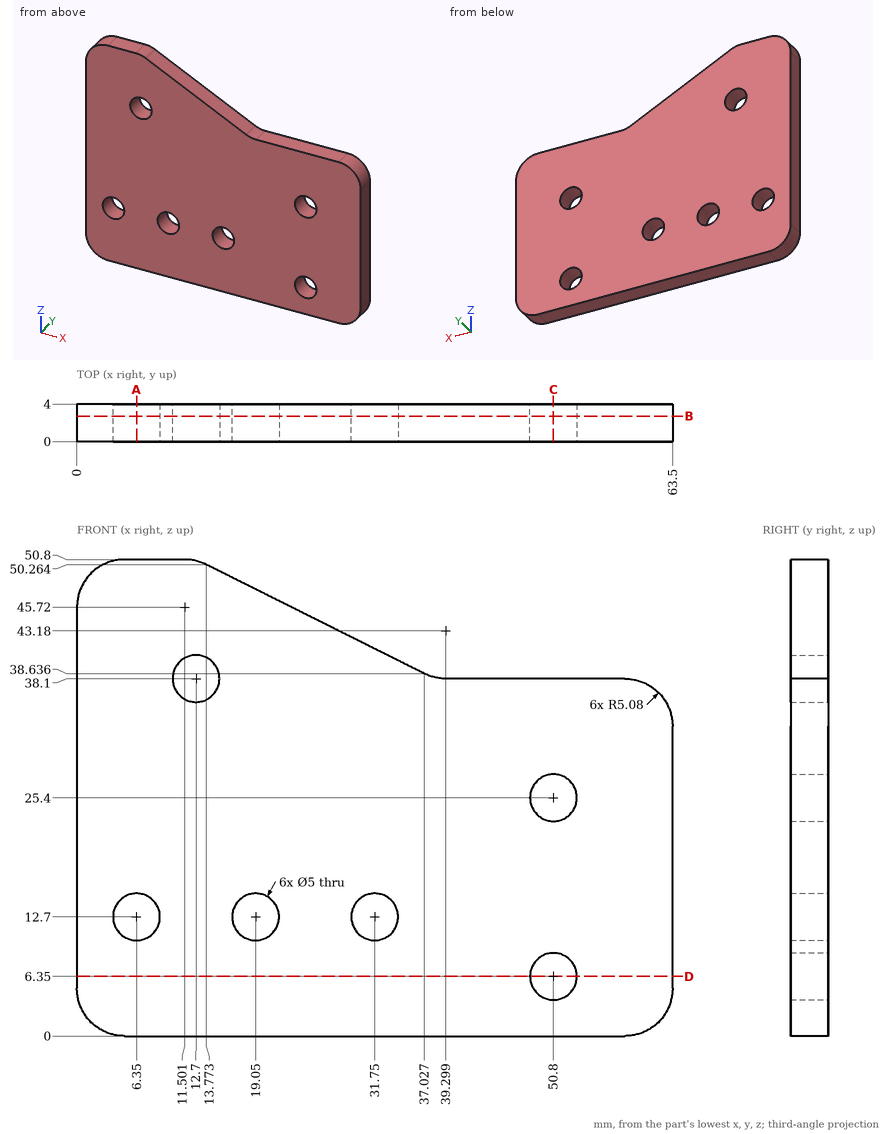
Geometry check sheet. Reference: drawing and pictorial views, mm from the part's lowest x, y, z. Give positions to 0.01 mm unless a question says otherwise; leave off trailing zeros. Order: outer loops, then holes, each group sorted by start corner. A loop starts at its lowest first (then second) coordinate and runs counter-clockwise, first axis right, second up. Notation, with made-up numbers: (-30.75, 61) -> (2.25, 61) arc R24 ccw to (2.25, 75) -> close; hole circle Ø5 at (39.25, 77). An arc over 180 degrees is marked (long way). Write each question's results on one line, items separated by ' | '. Start each with the question number.
(1) Scan lines: line 1 (Z direction, x = 50.8, y = 2.05); line 2 (X direction, y = 1.4, z = 25.5); line 3 (X direction, y = 3.35, z = 10.5) (1 decimal). Record each from-to range of solid material in increasing order.
(2) Sectioned sample at D-D (z = 6.35). Enter the section's corners in (x, y).
(3) Sectioned sample at B-B (y = 2.7). Enter the section's corners in (x, z).
(4) Sectioned sample at A-A (x = 6.35). Enter the section's corners in (y, z), plus the area to 3 significant figures.
(5) Sectioned sample at C-C (x = 50.8). Enter the section's corners in (y, z), plus the area to 3 significant figures.
Answer below:
1) line 1: 0 to 3.85, 8.85 to 22.9, 27.9 to 38.1 | line 2: 0 to 48.3, 53.3 to 63.5 | line 3: 0 to 5.2, 7.5 to 17.9, 20.2 to 30.6, 32.9 to 63.5
2) outline: (0, 0) -> (48.3, 0) -> (48.3, 4) -> (0, 4) -> close; (53.3, 0) -> (63.5, 0) -> (63.5, 4) -> (53.3, 4) -> close
3) outline: (0, 5.08) arc R5.08 ccw to (5.08, 0) -> (58.42, 0) arc R5.08 ccw to (63.5, 5.08) -> (63.5, 33.02) arc R5.08 ccw to (58.42, 38.1) -> (39.3, 38.1) arc R5.08 cw to (37.03, 38.64) -> (13.77, 50.26) arc R5.08 ccw to (11.5, 50.8) -> (5.08, 50.8) arc R5.08 ccw to (0, 45.72) -> close; hole circle Ø5 at (6.35, 12.7); hole circle Ø5 at (12.7, 38.1); hole circle Ø5 at (19.05, 12.7); hole circle Ø5 at (31.75, 12.7); hole circle Ø5 at (50.8, 6.35); hole circle Ø5 at (50.8, 25.4)
4) outline: (0, 0) -> (4, 0) -> (4, 10.2) -> (0, 10.2) -> close; (0, 15.2) -> (4, 15.2) -> (4, 50.8) -> (0, 50.8) -> close | area: 183 mm2
5) outline: (0, 0) -> (4, 0) -> (4, 3.85) -> (0, 3.85) -> close; (0, 8.85) -> (4, 8.85) -> (4, 22.9) -> (0, 22.9) -> close; (0, 27.9) -> (4, 27.9) -> (4, 38.1) -> (0, 38.1) -> close | area: 112 mm2
